Design review of the part shown in the three views and the two pictorial views. Dimensions are in mm from the part's minimum x, y and z. A direction names the side the tool comes from. Coordinates: 2 decimals unless noted, no trailing zeros. Order: outer loops, then holes, each group sorted by start corner. A loop starts at its lowest first (then second) coordinate and runs counter-clockwise, first axis right, second up. Notation, with made-up numbers: (17.5, 46) -> (22.5, 46) arc R26 cw to (22.5, 65) -> close; hole circle Ø9 at (79.25, -13). An arc over 180 degrees is marked (long way). Answer as a JSON object with one key per item and string values. Group by question number.
1) Wall thickness on L1, parallel to X at y = 0.65, z = 6.5 (1 decimal); L2, parallel to X at y = 0.95, z = 3.75 (1 decimal); L3, parallel to X at y = 2.75, z = 5.25 (1 decimal): over which ranges is each line inside the solid? List them lowest first.
2) Add section D-D, the plane y = 0.9. Write out the cut boundary in (x, z).
3) For pin 1 (1.5 mm diameter, centred on y = 3, z = 1.5, fed in from -X); pin 2 (1.5 mm diameter, centred on y = 2.5, z = 6.5, fed in from +X); pin 3 (1 mm diameter, centred on x = 11, z = 5, fed in from -Y) (1 decimal); pin 4 (4 mm diameter, centred on x = 13.01, z = 4, fed in from -Y), all flat-tipped, find the tip position at first contact; note any pin that passes through.
4) Machinability: for the marked faces 1 and 2, which of the approach directions +Z, -Z, +X, -X, +Y, -Y give a long, thin tool a straight path to every point of the face, cutting with its end or side? Answer none if there is none.
5) Add section B-B, the plane z = 4. Write out the cut boundary in (x, y).
6) Add section C-C, the plane y = 3.05. Write out the cut boundary in (x, z).
7) Draft analysis for pull direction X (two halves, no side actions). For the marked faces 3, 4, 5 and 6, state which applies: +X half, -X half, draft (parallel to the pull), parting line (faces both ways), or undercut.
8) Add section A-A, the plane y = 3.7. Write out the cut boundary in (x, z).
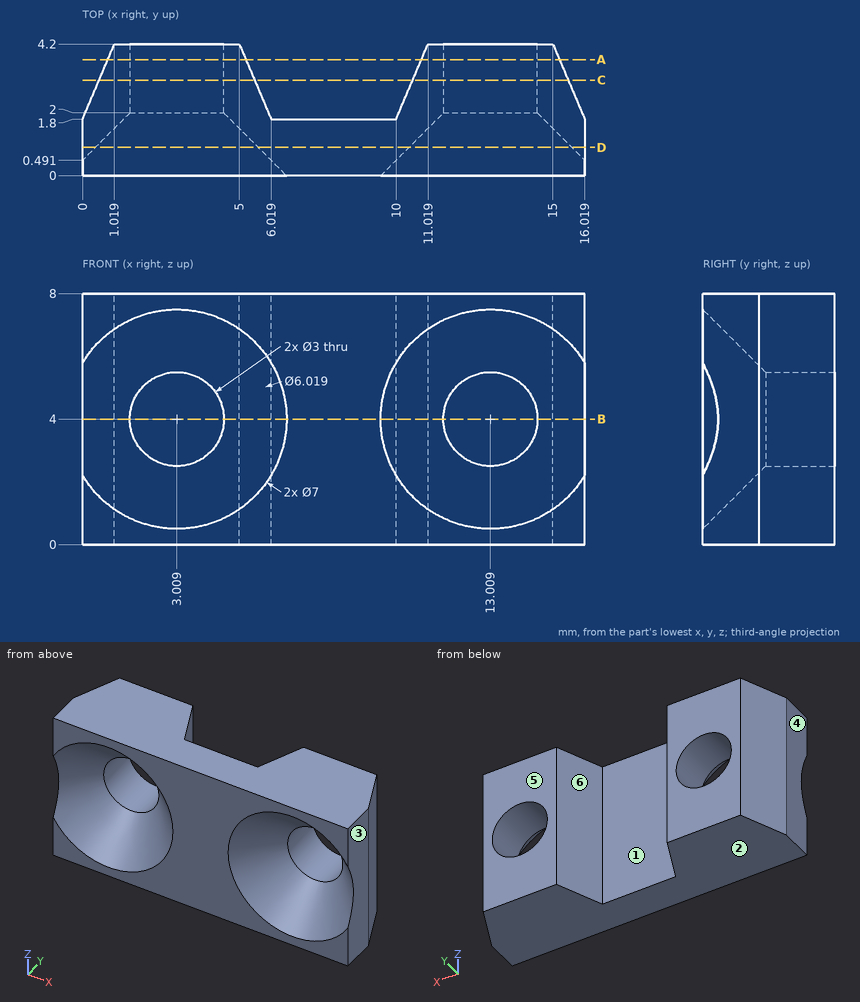
Output values:
{
 "1": {"L1": "x = 0 to 1.6, 4.4 to 11.6, 14.4 to 16", "L2": "x = 0 to 0.5, 5.5 to 10.5, 15.5 to 16", "L3": "x = 0.4 to 2.2, 3.8 to 5.6, 10.4 to 12.2, 13.8 to 15.6"},
 "2": {"outline": "(0, 0) -> (16.02, 0) -> (16.02, 8) -> (0, 8) -> close; hole circle Ø5.2 at (3.01, 4); hole circle Ø5.2 at (13.01, 4)"},
 "3": {"pin 1": "stops at x = 0.19", "pin 2": "stops at x = 16.02", "pin 3": "stops at y = 0.8", "pin 4": "stops at y = 1.5"},
 "4": {"face 1": "+Z, -Z, +Y", "face 2": "-Z, +X, -X, +Y, -Y"},
 "5": {"outline": "(0, 0.49) -> (1.51, 2) -> (1.51, 4.2) -> (1.02, 4.2) -> (0, 1.8) -> close; (4.51, 2) -> (6.51, 0) -> (9.51, 0) -> (11.51, 2) -> (11.51, 4.2) -> (11.02, 4.2) -> (10, 1.8) -> (6.02, 1.8) -> (5, 4.2) -> (4.51, 4.2) -> close; (14.51, 2) -> (16.02, 0.49) -> (16.02, 1.8) -> (15, 4.2) -> (14.51, 4.2) -> close"},
 "6": {"outline": "(0.53, 0) -> (5.49, 0) -> (5.49, 8) -> (0.53, 8) -> close; (10.53, 0) -> (15.49, 0) -> (15.49, 8) -> (10.53, 8) -> close; hole circle Ø3 at (3.01, 4); hole circle Ø3 at (13.01, 4)"},
 "7": {"face 3": "+X half", "face 4": "-X half", "face 5": "draft", "face 6": "undercut"},
 "8": {"outline": "(0.81, 0) -> (5.21, 0) -> (5.21, 8) -> (0.81, 8) -> close; (10.81, 0) -> (15.21, 0) -> (15.21, 8) -> (10.81, 8) -> close; hole circle Ø3 at (3.01, 4); hole circle Ø3 at (13.01, 4)"}
}
